Geometry: final body of the model. Coordinates: model frame, mm. Face numbers are marked on the shaded views. Round coordinates to 2 decimals unless told otherwise and drop trailing zeros. Loops run counter-clockwise (first coordinate to the right, second up) from the corner with the lowest first, then second, coordinate; pieces in that order, holes last. Notation, with made-up numbers: (44, -2) - (99, -2) arc R16 ccw to (99, 26) - close; hole circle Ø3 at (74.25, 88.25). An arc over 180 degrees is marked (long way). Return JSON: item names as keys, results as strings. Group by question number.
1. Section B-B on y = 3.5. Return loops of the section in (x, z).
2. Section C-C on x = -6. Return loops of the section in (y, z).
3. Material intervals for probe 1 along Y at (x, z) = (2, 1.3); probe 2 along Y at (x, z) = (5.75, 1.1); probe 3 along Y at (x, z) = (0, 0.3), sorted ascending.
4. Draft query along Y for the marked faces 1 and 2. Return one class per face: +Y half, -Y half, draft (parallel to the pull), parting line (faces both ways), or undercut.
5. Section A-A on z = 0.6. Return loops of the section in (x, y), and give its area (3 significant figures).
6. First-contact query: pin 1 Ø0.5 at (x, z) = (8.5, -0.5) entering from -Y; pin 2 Ø0.5 at (y, z) = (-1.5, 1.5) entering from +X; pin 3 Ø1.5 at (x, y) = (0, 0.5) entering from +Z; pin 4 Ø0.5 at (x, z) = (-6, 1.5) entering from +Y. Flat tips, straight axial feed; report the tip coordinate or a pass-through.
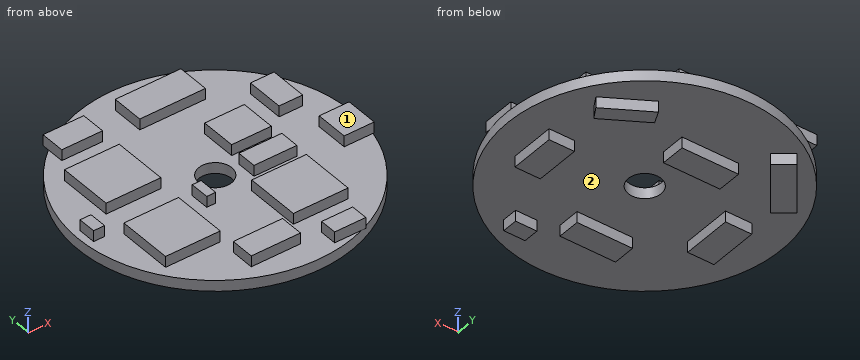
from build123d import *

# Parameters (mm, degrees)
F0_R     = 12.5
F1_DEPTH = 1
F2_W     = 5
F2_H     = 5
F2_W_2   = 3.627453
F2_H_2   = 3.235293
F2_W_3   = 6
F2_H_3   = 2.941177
F2_W_4   = 2.745098
F2_H_4   = 3
F2_W_5   = 3.72549
F2_H_5   = 2.254901
F2_W_6   = 4.502999
F2_H_6   = 2.156863
F2_W_7   = 2.843137
F2_H_7   = 1.568628
F2_W_8   = 2.156863
F2_H_8   = 3.431373
F2_W_9   = 3.921569
F2_H_9   = 1.808301
F2_W_10  = 1.00111
F2_H_10  = 1.626806
F2_W_11  = 0.813403
F2_H_11  = 1.751944
F3_DEPTH = 1
F4_W     = 2.405281
F4_H     = 4.543311
F4_W_2   = 5.166902
F4_H_2   = 2.227113
F4_W_3   = 2.316197
F4_H_3   = 4.097889
F4_W_4   = 5.077818
F4_H_4   = 2.048944
F4_W_5   = 1.95986
F4_H_5   = 1.425353
F5_DEPTH = 1
F7_D     = 3


with BuildPart() as f1:
    # F0 (on Top) → F1 (new body)
    with BuildSketch(Plane.XY):
        Circle(F0_R)
    extrude(amount=F1_DEPTH)

    # F2 (on face) → F3 (join)
    with BuildSketch(Plane.XY.offset(1)):
        with Locations((-7.002999, -4.014183)):
            Rectangle(F2_W, F2_H)
        with Locations((3.487197, -5.58281)):
            Rectangle(F2_W, F2_H)
        with Locations((-6.610843, 3.632876)):
            Rectangle(F2_W, F2_H)
        with Locations((4.173471, 2.750522)):
            Rectangle(F2_W_2, F2_H_2)
        with Locations((1.889157, 9.074051)):
            Rectangle(F2_W_3, F2_H_3)
        with Locations((10.872549, -1.5)):
            Rectangle(F2_W_4, F2_H_4)
        with Locations((-5.973588, 9.260326)):
            Rectangle(F2_W_5, F2_H_5)
        with Locations((-2.251499, -9.161241)):
            Rectangle(F2_W_6, F2_H_6)
        with Locations((3.467588, -10.867124)):
            Rectangle(F2_W_7, F2_H_7)
        with Locations((8.967588, 4.417189)):
            Rectangle(F2_W_8, F2_H_8)
        with Locations((4.124451, -0.90415)):
            Rectangle(F2_W_9, F2_H_9)
        with Locations((-11.311609, -0.098308)):
            Rectangle(F2_W_10, F2_H_10)
        with Locations((-2.395462, -1.787683)):
            Rectangle(F2_W_11, F2_H_11)
    extrude(amount=F3_DEPTH)

    # F4 (on face) → F5 (join)
    with BuildSketch(Plane(origin=(0, 0, 0), x_dir=(1, 0, 0), z_dir=(0, 0, -1))):
        with Locations((-7.670486, 1.073175)):
            Rectangle(F4_W, F4_H)
        with Locations((-1.211858, -5.162741)):
            Rectangle(F4_W_2, F4_H_2)
        with Locations((8.498355, 0.850464)):
            Rectangle(F4_W_3, F4_H_3)
        with Locations((-0.45464, 6.418247)):
            Rectangle(F4_W_4, F4_H_4)
        with Locations((4.756806, 8.689903)):
            Rectangle(F4_W_5, F4_H_5)
        Polygon((8.58744, -5.162742), (4.756805, -7.434397), (5.306815, -8.613397), (9.247805, -6.276298), align=None)
        Polygon((-4.953409, -8.613397), (-8.427706, -4.049185), (-9.972012, -5.162742), (-6.467846, -9.766193), align=None)
    extrude(amount=F5_DEPTH)

    # F7 (through all)
    with Locations(Plane.XY.offset(1)):
        with Locations((0, 0)):
            Hole(F7_D / 2)


solid = f1.part
Taken from the geometry:
{
 "1": {"outline": "(-12, 0) - (12, 0) - (12, 1) - (10.05, 1) - (10.05, 2) - (7.89, 2) - (7.89, 1) - (5.99, 1) - (5.99, 2) - (2.36, 2) - (2.36, 1) - (-4.11, 1) - (-4.11, 2) - (-9.11, 2) - (-9.11, 1) - (-12, 1) - close"},
 "2": {"outline": "(-10.97, 0) - (7.24, 0) - (7.24, -1) - (9.41, -1) - (9.41, 0) - (10.97, 0) - (10.97, 1) - (10.39, 1) - (10.39, 2) - (8.13, 2) - (8.13, 1) - (6.13, 1) - (6.13, 2) - (1.13, 2) - (1.13, 1) - (-1.51, 1) - (-1.51, 2) - (-6.51, 2) - (-6.51, 1) - (-10.97, 1) - close"},
 "3": {"probe 1": "-8.08 to -3.08, 7.6 to 10.54", "probe 2": "-8.08 to -3.08, -1.81 to 0, 1.13 to 4.37", "probe 3": "-12.5 to -1.5, 1.5 to 12.5"},
 "4": {"face 1": "draft", "face 2": "undercut"},
 "5": {"outline": "circle Ø25 at (0, 0); hole circle Ø3 at (0, 0)", "area": "484 mm2"},
 "6": {"pin 1": "y = -2.9", "pin 2": "x = 12.25", "pin 3": "through", "pin 4": "y = 10.39"}
}
